Build history of the part. All positions in model axes, mm. A direction names the side the tool comes from. Round coordinates to 2 decimals unless told otherwise and drop trailing zeros. Loops run counter-clockwise (first coordinate to the right, second up) from the corner with the lowest first, then second, coordinate; pieces in that order, holes last. Notation, with made-up numbers: (47.25, -5.75) - (100.25, -5.75) arc R28 ccw to (100.25, 19.25) - close; hole circle Ø5 at (40.25, 12.25). An arc over 180 degrees is marked (long way). Use a Markdown table: item, result.
Autodesk Inventor part; units mm, degrees
ref_plane "YZ Plane" through (0, 0, 0) normal (1, 0, 0) x (0, 1, 0)
ref_plane "XZ Plane" through (0, 0, 0) normal (0, 1, 0) x (-1, 0, 0)
ref_plane "XY Plane" through (0, 0, 0) normal (0, 0, 1) x (1, 0, 0)
sketch "Sketch1" plane through (0, 0, 0) normal (0, 0, 1) x (1, 0, 0)
  line L0 (0, 0) -> (-188.3663, 0)
  line L1 (-188.3663, 0) -> (-188.3663, -1500)
  line L2 (-188.3663, -1500) -> (0, -1500)
  line L3 (0, -1500) -> (0, 0)
  line L4 (-188.3663, -1400) -> (-81, -1400)
  line L5 (-81, -1400) -> (-81, -1394)
  line L6 (-81, -1394) -> (-188.3663, -1394)
  line L7 (-188.3663, -1394) -> (-188.3663, -1400)
  line L8 (-188.3663, -900) -> (-81, -900)
  line L9 (-81, -900) -> (-81, -894)
  line L10 (-81, -894) -> (-188.3663, -894)
  line L11 (-188.3663, -894) -> (-188.3663, -900)
  line L12 (-188.3663, -400) -> (-81, -400)
  line L13 (-81, -400) -> (-81, -394)
  line L14 (-81, -394) -> (-188.3663, -394)
  line L15 (-188.3663, -394) -> (-188.3663, -400)
  dimension "d0" = 1500
  dimension "d1" = 188.3663
  dimension "d2" = 6
  dimension "d4" = 100
  dimension "d7" = 500
  dimension "d23" = 81
extrude "Plate1" add sketch "Sketch1" along normal blind 4 contours L3 L2 L1 L4 L5 L6 L8 L9 L10 L12 L13 L14 L0
sketch "Sketch2" plane through (4, 0, 0) normal (-1, 0, 0) x (0, -1, 0)
  line L0 (1500, 0) -> (0, 0)
  line L1 (0, 0) -> (0, 35)
  line L2 (0, 35) -> (1500, 35)
  line L3 (1500, 35) -> (1500, 0)
edge flange "Flange1" height 35 angle 90 thickness 4 bend radius 4 thickness toward (-1, 0, 0) relief tear relief width 4 relief depth 2 edges at (0, -750, 4) wall of the first edge with corners at (4, -1500, 0) (4, 0, 0) (4, 0, 35) (4, -1500, 35)
bend "Bend1"
corner "Corner1"
equation "\"d1\" = Stringer1_deep"
equation "\"d12\" = Thickness"
equation "\"d13\" = BendReliefWidth"
equation "\"d14\" = BendReliefDepth"
equation "\"d15\" = MinimumRemnant"
equation "\"d16\" = TransitionRadius"
equation "\"d19\" = BendRadius"
equation "\"d20\" = CornerReliefSize"
equation "\"d21\" = GapSize"
equation "\"d22\" = JacobiRadiusSize"
equation "\"BendRadius\" = Thickness"
equation "\"BendReliefWidth\" = Thickness"
equation "\"BendReliefDepth\" = 0.5 * Thickness"
equation "\"CornerReliefSize\" = 4 * Thickness"
equation "\"MinimumRemnant\" = 2 * Thickness"
equation "\"TransitionRadius\" = BendRadius"
equation "\"JacobiRadiusSize\" = BendRadius"
equation "\"GapSize\" = Thickness"
equation "\"Stringer1_deep\" = 188.36631"
properties part number "01.3 GBK stringer" material "Steel"
Q1. Which spindle directions (+Z, -Z, +X, -X, +Y, -Y) get a long thin tool onto all of the face, cutting with end or side? Do faces 1 (the face through (-97, -740, 0)), 2 (the face through (-97, -740, 4)). Say none if no direction does.
Results found:
| item | result |
|---|---|
| face 1 | -Z, +X, -X, +Y, -Y |
| face 2 | +Z, -X, +Y, -Y |
Q2. Cut at B-B, the plane y = -1189.5. List the corners of the cut face in (x, z), plus the area to 3 significant figures.
Results found:
| item | result |
|---|---|
| outline | (-188.37, 0) - (-4, 0) arc R8 ccw to (4, 8) - (4, 35) - (0, 35) - (0, 8) arc R4 cw to (-4, 4) - (-188.37, 4) - close |
| area | 883 mm2 |
Q3. Cut at C-C, the plane z = 28.5. List the corners of the cut face in (x, y), plus the area to 3 significant figures.
Results found:
| item | result |
|---|---|
| outline | (0, -1500) - (4, -1500) - (4, 0) - (0, 0) - close |
| area | 6,000 mm2 |
Q4. Probe line 1 (X direction, y = -810.5, z = 8.5). List the from-to ranges inside material, lowest first.
Results found:
| item | result |
|---|---|
| line 1 | x = 0 to 4 |
Q5. Cut at A-A, the plane x = -104.5. List the corners of the cut face in (y, z).
Results found:
| item | result |
|---|---|
| outline | (-1500, 0) - (-1400, 0) - (-1400, 4) - (-1500, 4) - close; (-1394, 0) - (-900, 0) - (-900, 4) - (-1394, 4) - close; (-894, 0) - (-400, 0) - (-400, 4) - (-894, 4) - close; (-394, 0) - (0, 0) - (0, 4) - (-394, 4) - close |
Q6. Drop flat-ended pins along their axis: pin 1 (5 mm diameter, centred on x = -121, y = -441.5, fed in from +Z); pin 2 (12 mm diameter, centred on y = -655, z = 26, fed in from -X); pin 3 (1.2 mm diameter, centred on y = -896, z = 1, fed in from -X); pin 4 (12 mm diameter, centred on x = -76.5, z = 12, fed in from -Y). Give the stop position or say it passes through.
Results found:
| item | result |
|---|---|
| pin 1 | stops at z = 4 |
| pin 2 | stops at x = 0 |
| pin 3 | stops at x = -81 |
| pin 4 | passes through |
Q7. Cut at D-D, the plane x = -48.5. List the corners of the cut face in (y, z), plus the area to 3 significant figures.
Results found:
| item | result |
|---|---|
| outline | (-1500, 0) - (0, 0) - (0, 4) - (-1500, 4) - close |
| area | 6,000 mm2 |
